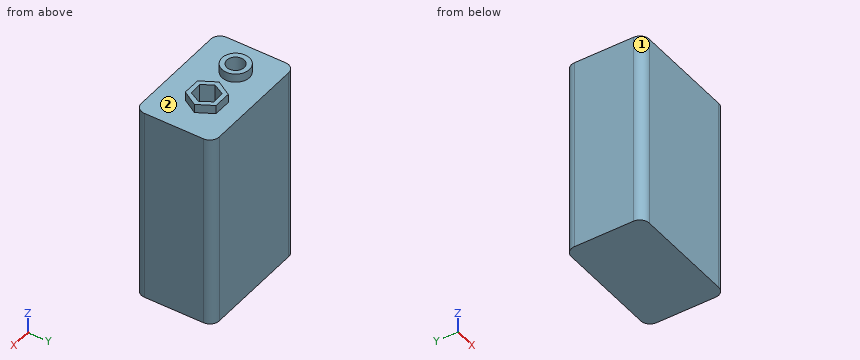
from build123d import *

# Parameters (mm, degrees)
F0_W     = 39.259444
F0_H     = 63.933932
F1_DEPTH = 25.4
F2_R     = 3.066051
F3_R     = 4.474413
F4_DEPTH = 34.798
F6_DEPTH = 34.798
F7_R     = 2.859954
F8_DEPTH = 35.306


with BuildPart() as f1:
    # F0 (on Front) → F1 (new body)
    with BuildSketch(Plane.XZ):
        Rectangle(F0_W, F0_H)
    extrude(amount=F1_DEPTH)

    # F2
    f2_edges = [f1.edges().sort_by_distance(p)[0] for p in [
        (-19.629722, -25.4, 0),
        (19.629722, 0, 0),
        (19.629722, -25.4, 0),
        (-19.629722, 0, 0),
    ]]
    fillet(f2_edges, radius=F2_R)

    # F3 (on Top) → F4 (join)
    with BuildSketch(Plane.XY):
        with Locations((-8.871355, -11.997017)):
            Circle(F3_R)
    extrude(amount=F4_DEPTH)

    # F5 (on Top) → F6 (join)
    with BuildSketch(Plane.XY):
        Polygon((2.987864, -16.336561), (8.799858, -16.389728), (11.751899, -11.382976), (8.891946, -6.323057), (3.079951, -6.269891), (0.12791, -11.276643), align=None)
    extrude(amount=F6_DEPTH)

    # F7 (on Top) → F8 (cut)
    with BuildSketch(Plane.XY):
        with Locations((-8.799859, -11.989804)):
            Circle(F7_R)
        Polygon((7.888282, -7.664617), (3.739939, -7.809872), (1.791562, -11.475069), (3.991527, -14.995012), (8.13987, -14.849758), (10.088247, -11.18456), align=None)
    extrude(amount=F8_DEPTH, mode=Mode.SUBTRACT)


solid = f1.part
Model file for the job. Use its own axes, mm. Face numbers are marked on the shaded views. A direction names the side the tool comes from. Round coordinates to 2 decimals unless told otherwise and drop trailing zeros. Order: outer loops, then holes, each group sorted by start corner. A loop starts at its lowest first (then second) coordinate and runs counter-clockwise, first axis right, second up.
(1) Drill centre lines: line 1 (X direction, y = -14.25, z = 21); line 2 (Z direction, x = -16.5, y = -13); line 3 (Y direction, x = 4, z = 10). Where is each one in solid material? Low to high.
(2) Band-saw the part on C-C (y = -20). List the corners of the cut face in (x, z).
(3) Band-saw the part on A-A (z = 17.5). List the corners of the cut face in (x, y), then the cut area to 3 significant figures.
(4) 3-axis set-ups, long thin cutter, end or side, ignore diameter. For the marked faces 1 and 2: which of +Z, -Z, +X, -X, +Y, -Y reach the whole face in a straight line?
(5) Band-saw the part on D-D (x = 6.5). List the corners of the cut face in (y, z).
(6) Pin check, flat tips, straight feed: pin 1 (2 mm diameter, centred on x = 4.5, y = -12.5, fed in from +Z); pin 2 (7.5 mm diameter, centred on x = -3.5, y = -17.5, fed in from +Z); pin 3 (1.5 mm diameter, centred on x = 14.5, y = -2.5, fed in from +Z). Stop position of each tip, or through.
(7) Band-saw the part on B-B (x = -2). List the corners of the cut face in (y, z).
Verdict:
1. line 1: x = -19.63 to -10.55, -7.05 to 3.53, 8.46 to 19.63
1. line 2: z = -31.97 to 31.97
1. line 3: y = -25.4 to -14.99, -7.8 to 0
2. outline: (-19.63, -31.97) - (19.63, -31.97) - (19.63, 31.97) - (-19.63, 31.97) - close
3. outline: (-19.63, -22.33) arc R3.07 ccw to (-16.56, -25.4) - (16.56, -25.4) arc R3.07 ccw to (19.63, -22.33) - (19.63, -3.07) arc R3.07 ccw to (16.56, 0) - (-16.56, 0) arc R3.07 ccw to (-19.63, -3.07) - close; hole circle Ø5.72 at (-8.8, -11.99); hole (1.79, -11.48) - (3.99, -15) - (8.14, -14.85) - (10.09, -11.18) - (7.89, -7.66) - (3.74, -7.81) - close
3. area: 919 mm2
4. face 1: +Z, -Z, -X, -Y
4. face 2: +Z
5. outline: (-25.4, -31.97) - (0, -31.97) - (0, 31.97) - (-6.3, 31.97) - (-6.3, 34.8) - (-7.71, 34.8) - (-7.71, 0) - (-14.91, 0) - (-14.91, 34.8) - (-16.37, 34.8) - (-16.37, 31.97) - (-25.4, 31.97) - close
6. pin 1: stops at z = 0
6. pin 2: stops at z = 34.8
6. pin 3: stops at z = 31.97
7. outline: (-25.4, -31.97) - (0, -31.97) - (0, 31.97) - (-25.4, 31.97) - close
